from build123d import *

# Parameters (mm, degrees)
SKETCH1_W           = 170
SKETCH1_H           = 146
BOSS_EXTRUDE1_DEPTH = 103
SKETCH2_R           = 65
BOSS_EXTRUDE2_DEPTH = 113.2
SKETCH3_R           = 73
BOSS_EXTRUDE3_DEPTH = 169.8


with BuildPart() as part:
    # Sketch1 → Boss-Extrude1 (new body)
    with BuildSketch(Plane.XY):
        Rectangle(SKETCH1_W, SKETCH1_H)
    extrude(amount=BOSS_EXTRUDE1_DEPTH)

    # Sketch2 → Boss-Extrude2 (add)
    with BuildSketch(Plane.XY.offset(103)):
        Circle(SKETCH2_R)
    extrude(amount=BOSS_EXTRUDE2_DEPTH)

    # Sketch3 → Boss-Extrude3 (add)
    with BuildSketch(Plane.XY.offset(216.2)):
        Circle(SKETCH3_R)
    extrude(amount=BOSS_EXTRUDE3_DEPTH)


solid = part.part
Work out the finished part from the listing and answer in its coordinate system (mm). A direction names the side the tool comes from. Give positions to 0.01 mm unless a question says otherwise; leave off trailing zeros. Loops run counter-clockwise (first coordinate to the right, second up) from the corner with the lowest first, then second, coordinate; pieces in that order, holes last. Notation, with made-up numbers: (29, 64) -> (88, 64) arc R24 cw to (88, 75) -> close; hole circle Ø3 at (-22.75, 64). An arc over 180 degrees is marked (long way). Use a Markdown table: item, result. Add a question column.
1) Each of these flat-tipped pins is pushed along its axis until it touches: P1, Ø1, axis at x = 2.5, y = -52, coming from the -Z side; P2, Ø5, axis at y = -5.5, z = 223, coming from the +X side; P3, Ø4, axis at x = 56.5, z = 338, coming from the +Y side; P4, Ø1.5, axis at x = -3, z = 197, coming from the -Y side. Where does it stop, or does it pass through?
2) The part is cut by section B-B, the plane x = 0. Determine the outline of the cut face in (y, z), plus the area to 3 significant figures.
3) Which of the six approach directions +Z, -Z, +X, -X, +Y, -Y give full straight-line access (tool end or side, diameter ignored) to faces 4 (the cylindrical face through (62, 19.52, 158.81)), 5 (the flat face through (-1, 1, 0)), 6 (the cylindrical face through (-15.825, -71.264, 299.911))?
4) The part is cut by section C-C, the plane z = 267.5. Determine the outline of the cut face in (x, y), plus the area to 3 significant figures.
5) For a pull along Z with two mould halves and no side action, classify faces 1 (the flat face through (-1, 1, 386)), 2 (the flat face through (-49, -43, 216.2)), 3 (the flat face through (-1, 73, 51)) as +Z half, -Z half, draft (parallel to the pull), parting line (faces both ways), or undercut.
6) Consider line 1 along Z through (x, y) = (44, -50); line 2 along Y through (x, z) = (0.5, 322.5); line 3 along Z through (x, y) = (77, 26.5). Determine where each line is inside the solid, lowest interval first.
7) The part is cut by section A-A, the plane y = 0. Determine the outline of the cut face in (x, z), plus the area to 3 significant figures.
Reported:
| question | item | result |
|---|---|---|
| 1 | P1 | stops at z = 0 |
| 1 | P2 | stops at x = 72.94 |
| 1 | P3 | stops at y = 48.57 |
| 1 | P4 | stops at y = -64.96 |
| 2 | outline | (-73, 0) -> (73, 0) -> (73, 103) -> (65, 103) -> (65, 216.2) -> (73, 216.2) -> (73, 386) -> (-73, 386) -> (-73, 216.2) -> (-65, 216.2) -> (-65, 103) -> (-73, 103) -> close |
| 2 | area | 54,500 mm^2 |
| 3 | face 4 | none |
| 3 | face 5 | -Z, +X, -X, +Y, -Y |
| 3 | face 6 | +Z |
| 4 | outline | circle Ø146 at (0, 0) |
| 4 | area | 16,700 mm^2 |
| 5 | face 1 | +Z half |
| 5 | face 2 | undercut |
| 5 | face 3 | draft |
| 6 | line 1 | z = 0 to 103, 216.2 to 386 |
| 6 | line 2 | y = -73 to 73 |
| 6 | line 3 | z = 0 to 103 |
| 7 | outline | (-85, 0) -> (85, 0) -> (85, 103) -> (65, 103) -> (65, 216.2) -> (73, 216.2) -> (73, 386) -> (-73, 386) -> (-73, 216.2) -> (-65, 216.2) -> (-65, 103) -> (-85, 103) -> close |
| 7 | area | 57,000 mm^2 |
